```python
from build123d import *

# Parameters (mm, degrees)
SKETCH1_W           = 38
SKETCH1_H           = 36
SKETCH1_R           = 1.55
SKETCH1_R_2         = 11.5
BOSS_EXTRUDE1_DEPTH = 5
SKETCH2_W           = 38
SKETCH2_H           = 4.5
BOSS_EXTRUDE2_DEPTH = 20
SKETCH3_R           = 2.05
BOSS_EXTRUDE3_DEPTH = 5
BOSS_EXTRUDE4_START = -5
SKETCH4_W           = 57
SKETCH4_H           = 57
SKETCH4_R           = 2.5
SKETCH4_W_2         = 38
SKETCH4_H_2         = 45
SKETCH4_R_2         = 1.55
SKETCH4_R_3         = 11.5
BOSS_EXTRUDE4_DEPTH = 5
FILLET2_R           = 2
SKETCH6_R           = 19.25
CUT_EXTRUDE2_DEPTH  = 48.628772816
CUT_EXTRUDE3_DEPTH  = 5


with BuildPart() as part:
    # Sketch1 → Boss-Extrude1 (new body)
    with BuildSketch(Plane.XY):
        Rectangle(SKETCH1_W, SKETCH1_H)
        with Locations((15.5, 15.5)):
            Circle(SKETCH1_R, mode=Mode.SUBTRACT)
        with Locations((-15.5, 15.5)):
            Circle(SKETCH1_R, mode=Mode.SUBTRACT)
        with Locations((15.5, -15.5)):
            Circle(SKETCH1_R, mode=Mode.SUBTRACT)
        with Locations((-15.5, -15.5)):
            Circle(SKETCH1_R, mode=Mode.SUBTRACT)
        Circle(SKETCH1_R_2, mode=Mode.SUBTRACT)
    extrude(amount=BOSS_EXTRUDE1_DEPTH)

    # Sketch2 → Boss-Extrude2 (add)
    with BuildSketch(Plane.XY.offset(5)):
        with Locations((0, 20.25)):
            Rectangle(SKETCH2_W, SKETCH2_H)
        with Locations((0, -20.25)):
            Rectangle(SKETCH2_W, SKETCH2_H)
    extrude(amount=-BOSS_EXTRUDE2_DEPTH)

    # Sketch3 → Boss-Extrude3 (add)
    # profile 1 of 2: a face of its own
    with BuildSketch(Plane(origin=(0, 0, -15), x_dir=(-1, 0, 0), z_dir=(0, 0, -1))):
        with BuildLine():
            Line((-19, 26.367593747), (-19, 22.5))
            Line((-19, 22.5), (19, 22.5))
            Line((19, 22.5), (19, 26.367593747))
            ThreePointArc((19, 26.367593747), (9.982564879, 30.928924948), (-6e-09, 32.5))
            ThreePointArc((-6e-09, 32.5), (-9.982564884, 30.928924946), (-19, 26.367593747))
        make_face()
        with Locations((-8.80698434, 27.105110714)):
            Circle(SKETCH3_R, mode=Mode.SUBTRACT)
        with Locations((8.80698434, 27.105110714)):
            Circle(SKETCH3_R, mode=Mode.SUBTRACT)
    # profile 2 of 2: a face of its own
    with BuildSketch(Plane(origin=(0, 0, -15), x_dir=(-1, 0, 0), z_dir=(0, 0, -1))):
        with BuildLine():
            Line((-19, -22.5), (-19, -26.367593747))
            ThreePointArc((-19, -26.367593747), (-9.982564919, -30.928924935), (-7.8e-08, -32.5))
            ThreePointArc((-7.8e-08, -32.5), (9.982564844, -30.928924959), (19, -26.367593747))
            Line((19, -26.367593747), (19, -22.5))
            Line((19, -22.5), (-19, -22.5))
        make_face()
        with Locations((-8.80698434, -27.105110714)):
            Circle(SKETCH3_R, mode=Mode.SUBTRACT)
        with Locations((8.80698434, -27.105110714)):
            Circle(SKETCH3_R, mode=Mode.SUBTRACT)
    extrude(amount=-BOSS_EXTRUDE3_DEPTH)

    # Sketch4 → Boss-Extrude4 (add)
    # profile 1 of 6: a face of its own
    with BuildSketch(Plane.XY.offset(5).offset(BOSS_EXTRUDE4_START)):
        Rectangle(SKETCH4_W, SKETCH4_H)
        with Locations((-23.57, -23.57)):
            Circle(SKETCH4_R, mode=Mode.SUBTRACT)
        with Locations((23.57, -23.57)):
            Circle(SKETCH4_R, mode=Mode.SUBTRACT)
        Rectangle(SKETCH4_W_2, SKETCH4_H_2, mode=Mode.SUBTRACT)
        with Locations((-23.57, 23.57)):
            Circle(SKETCH4_R, mode=Mode.SUBTRACT)
        with Locations((23.57, 23.57)):
            Circle(SKETCH4_R, mode=Mode.SUBTRACT)
    # profile 2 of 6: a face of its own
    with BuildSketch(Plane.XY.offset(5).offset(BOSS_EXTRUDE4_START)):
        Rectangle(SKETCH4_W_2, SKETCH4_H_2)
        with Locations((-15.5, -15.5)):
            Circle(SKETCH4_R_2, mode=Mode.SUBTRACT)
        Circle(SKETCH4_R_3, mode=Mode.SUBTRACT)
        with Locations((15.5, -15.5)):
            Circle(SKETCH4_R_2, mode=Mode.SUBTRACT)
        with Locations((-15.5, 15.5)):
            Circle(SKETCH4_R_2, mode=Mode.SUBTRACT)
        with Locations((15.5, 15.5)):
            Circle(SKETCH4_R_2, mode=Mode.SUBTRACT)
    # profile 3 of 6: a face of its own
    with BuildSketch(Plane.XY.offset(5).offset(BOSS_EXTRUDE4_START)):
        with Locations((-15.5, 15.5)):
            Circle(SKETCH4_R_2)
    # profile 4 of 6: a face of its own
    with BuildSketch(Plane.XY.offset(5).offset(BOSS_EXTRUDE4_START)):
        with Locations((-15.5, -15.5)):
            Circle(SKETCH4_R_2)
    # profile 5 of 6: a face of its own
    with BuildSketch(Plane.XY.offset(5).offset(BOSS_EXTRUDE4_START)):
        with Locations((15.5, -15.5)):
            Circle(SKETCH4_R_2)
    # profile 6 of 6: a face of its own
    with BuildSketch(Plane.XY.offset(5).offset(BOSS_EXTRUDE4_START)):
        with Locations((15.5, 15.5)):
            Circle(SKETCH4_R_2)
    extrude(amount=BOSS_EXTRUDE4_DEPTH)

    # Fillet2
    fillet2_edges = [part.edges().sort_by_distance(p)[0] for p in [
        (28.5, -28.5, 2.5),
        (-28.5, -28.5, 2.5),
        (-28.5, 28.5, 2.5),
        (28.5, 28.5, 2.5),
    ]]
    fillet(fillet2_edges, radius=FILLET2_R)

    # Sketch6 → Cut-Extrude2 (cut, through all)
    with BuildSketch(Plane.XY.offset(5)):
        Circle(SKETCH6_R)
    extrude(amount=-CUT_EXTRUDE2_DEPTH, mode=Mode.SUBTRACT)

    # Sketch7 → Cut-Extrude3 (cut)
    with BuildSketch(Plane.XY.offset(5)):
        Polygon((18.5, 28.5), (-18.5, 28.5), (-12.5, 22.5), (12.5, 22.5), align=None)
        Polygon((-12.5, -22.5), (-18.5, -28.5), (18.5, -28.5), (12.5, -22.5), align=None)
    extrude(amount=-CUT_EXTRUDE3_DEPTH, mode=Mode.SUBTRACT)


solid = part.part
```
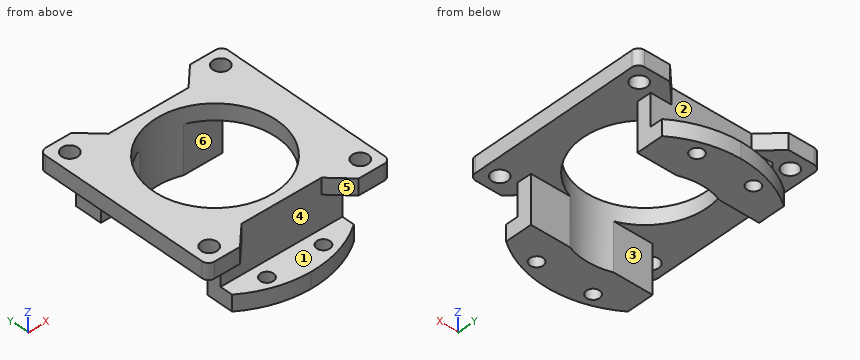
Here's how the part is built. I have some questions about the finished solid (model axes, mm). Face numbers are marked on the shaded views. A direction names the side the tool comes from. Coordinates: 2 decimals unless noted, no trailing zeros. Loops run counter-clockwise (first coordinate to the right, second up) from the corner with the lowest first, then second, coordinate; pieces in that order, holes last. Notation, with made-up numbers: (84.25, 3) - (101.25, 3) arc R24 ccw to (101.25, 38) - close; hole circle Ø5 at (-10, 26.5). An arc over 180 degrees is marked (long way). Answer as CSV lines item,"result".
Q1. For the marked faces 4, 5 and 6, which set-ups out of +Z, -Z, +X, -X, +Y, -Y let a thin tool reach every point of the face, with its end or its side?
Response:
face 4,"-Y"
face 5,"+Z, -Y"
face 6,"-Z, +X, -X"
Q2. If we section it at D-D, the plane y = -23.57: Write out the boundary of the cut face in (x, z), and give its area (3 significant figures).
Response:
outline,"(-28.5, 0) - (-26.07, 0) - (-26.07, 5) - (-28.5, 5) - close; (-21.07, 0) - (-13.57, 0) - (-13.57, 5) - (-21.07, 5) - close; (-19, -15) - (19, -15) - (19, -10) - (-19, -10) - close; (13.57, 0) - (21.07, 0) - (21.07, 5) - (13.57, 5) - close; (26.07, 0) - (28.5, 0) - (28.5, 5) - (26.07, 5) - close"
area,"289 mm2"
Q3. If we section it at A-A, the plane y = 0: Write out the boundary of the cut face in (x, z), and give its area (3 significant figures).
Response:
outline,"(-28.5, 0) - (-19.25, 0) - (-19.25, 5) - (-28.5, 5) - close; (19.25, 0) - (28.5, 0) - (28.5, 5) - (19.25, 5) - close"
area,"92.5 mm2"
Q4. If I drill on L1, parallel to Y at x = -3, z = -5.25; L2, parallel to Y at x = -0.5, z = -3.75; L3, parallel to Y at x = 23.57, z = 3.9, over which ranges is the centre line in solid material (lowest first)? Write a range as [from, to].
Response:
L1,"[-22.5, -19.01], [19.01, 22.5]"
L2,"[-22.5, -19.24], [19.24, 22.5]"
L3,"[-28.5, -26.07], [-21.07, 21.07], [26.07, 28.5]"
Q5. We'd pull the mould along Y, two halves only. Please class the marked faces 1, 2 and 3: pulls with the +Y half, pulls with the -Y half, needs draft (parallel to the pull), parting line crosses it, or undercut.
Response:
face 1,"needs draft"
face 2,"pulls with the +Y half"
face 3,"undercut"
Q6. For pin 1 (4 mm diameter, centred on y = 21.5, z = -8, fed in from +X); pin 2 (4 mm diameter, centred on y = -21, z = -6, fed in from -X); pin 3 (9.5 mm diameter, centred on x = -13.5, z = -9.5, fed in from +Y); pin 4 (4 mm diameter, centred on y = -21, z = -1, fed in from -X), each with a flat end and sliding along its axis, tell me the tip position at first contact or that it passes through.
Response:
pin 1,"x = 19"
pin 2,"x = -19"
pin 3,"y = 31.29"
pin 4,"x = -28.5"
Q7. If we section it at B-B, the plane z = -2.5: Write out the boundary of the cut face in (x, y).
Response:
outline,"(-19, -22.5) - (19, -22.5) - (19, -18) - (6.82, -18) arc R19.25 cw to (-6.82, -18) - (-19, -18) - close; (-19, 18) - (-6.82, 18) arc R19.25 cw to (6.82, 18) - (19, 18) - (19, 22.5) - (-19, 22.5) - close"
Q8. If we section it at C-C, the plane x = -23.57: Write out the boundary of the cut face in (y, z), and give its area (3 significant figures).
Response:
outline,"(-28.5, 0) - (-26.07, 0) - (-26.07, 5) - (-28.5, 5) - close; (-21.07, 0) - (21.07, 0) - (21.07, 5) - (-21.07, 5) - close; (26.07, 0) - (28.5, 0) - (28.5, 5) - (26.07, 5) - close"
area,"235 mm2"
